Study the drawing (mm; zero at the part's minimum x, y, z) and answer. Give positions to 0.01 mm unless a question says otherwise; leave off trailing zeros. Loops run counter-clockwise (first coordinate to the right, second up) from the corner with the lowest first, then second, coordinate; pieces in that order, holes last. Notation, with made-up numbers: M 59,13 L 118,13 A30 cw 118,44 Z; hole C 44,-37.75 d9. An arc over 180 degrees is marked long. Return JSON: item names as keys, results as strings.
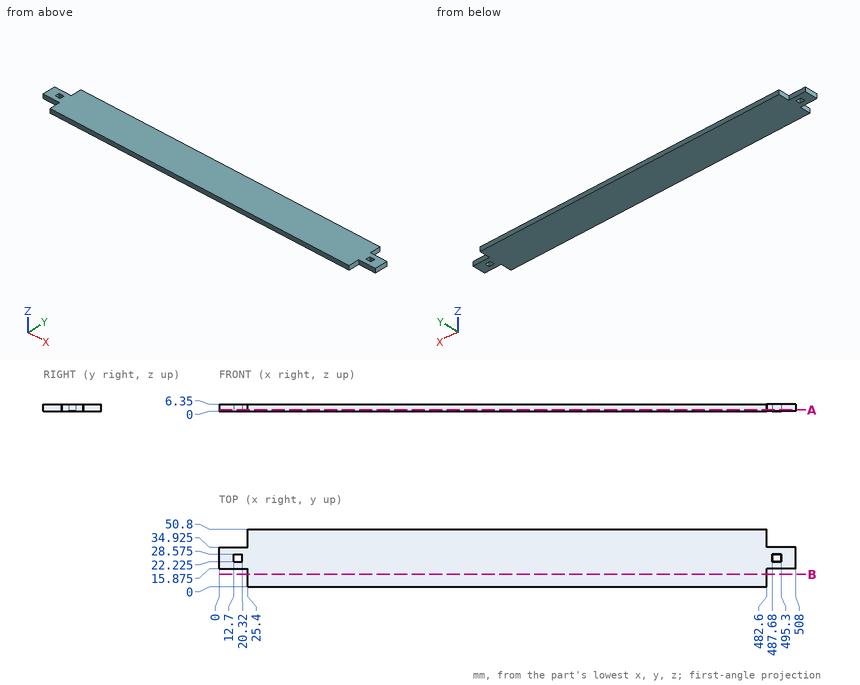
(1) Straight lines are drawn through the part: line 1 along X through (y, z) = (24.5, 4.25); line 2 along X through (y, z) = (47, 2.75). For each, find the intervals that lie inside material, in ascending order.
Values follow:
{"line 1": "0 to 12.7, 20.32 to 487.68, 495.3 to 508", "line 2": "25.4 to 482.6"}
(2) The part is cut by section A-A (z = 1.25). Determine the outline of the cut face in (x, y) (3 decimals).
Values follow:
{"outline": "M 0,15.875 L 25.4,15.875 L 25.4,0 L 482.6,0 L 482.6,15.875 L 508,15.875 L 508,34.925 L 482.6,34.925 L 482.6,50.8 L 25.4,50.8 L 25.4,34.925 L 0,34.925 Z; hole M 12.7,22.225 L 20.32,22.225 L 20.32,28.575 L 12.7,28.575 Z; hole M 487.68,22.225 L 495.3,22.225 L 495.3,28.575 L 487.68,28.575 Z"}
(3) Given pin 1 (1 mm diameter, centred on y = 41, z = 3, fed in from -X); pin 2 (1.9 mm diameter, centred on x = 15.5, z = 3, fed in from -Y) (3 decimals); pin 3 (1.9 mm diameter, centred on x = 15, z = 1.5, fed in from +Y) (3 decimals), each flat-ended and moving along its own axis, determine where each tip first touches the part or whether it passes through.
Values follow:
{"pin 1": "x = 25.4", "pin 2": "y = 15.875", "pin 3": "y = 34.925"}
(4) The part is cut by section B-B (y = 11). Determine the outline of the cut face in (x, z), and give its area (3 significant figures).
Values follow:
{"outline": "M 25.4,0 L 482.6,0 L 482.6,6.35 L 25.4,6.35 Z", "area": "2,900 mm²"}
